from build123d import *

# Parameters (mm, degrees)
CROQUIS1_R                                           = 42.5
CROQUIS1_R_2                                         = 12.5
SALIENTE_EXTRUIR1_DEPTH                              = 7
REFRENTADO_PARA_TORNILLO_TAP_N_CON_CABEZ_D           = 6.6
REFRENTADO_PARA_TORNILLO_TAP_N_CON_CABEZ_DEPTH       = 10
REFRENTADO_PARA_TORNILLO_TAP_N_CON_CABEZ_CSINK_D     = 13.44
REFRENTADO_PARA_TORNILLO_TAP_N_CON_CABEZ_CSINK_ANGLE = 90
REFRENTADO_PARA_TORNILLO_TAP_N_CON_CABEZ_TIP         = 1.982840043
REFRENTADO_PARA_TORNILLO_CON_CABEZA_TRON_D           = 3.4
REFRENTADO_PARA_TORNILLO_CON_CABEZA_TRON_DEPTH       = 10
REFRENTADO_PARA_TORNILLO_CON_CABEZA_TRON_CBORE_D     = 7
REFRENTADO_PARA_TORNILLO_CON_CABEZA_TRON_CBORE_DEPTH = 2.4
REFRENTADO_PARA_TORNILLO_CON_CABEZA_TRON_TIP         = 1.021463052


with BuildPart() as part:
    # Croquis1 → Saliente-Extruir1 (new body)
    with BuildSketch(Plane.XY):
        Circle(CROQUIS1_R)
        Circle(CROQUIS1_R_2, mode=Mode.SUBTRACT)
    extrude(amount=SALIENTE_EXTRUIR1_DEPTH)

    # Refrentado para tornillo tapón con cabeza plana de clavija de M61
    with Locations(Plane.XY.offset(7)):
        with Locations((0, 25), (17.67766953, 17.67766953), (25, 0), (17.67766953, -17.67766953), (0, -25), (-17.67766953, -17.67766953), (-25, 0), (-17.67766953, 17.67766953)):
            CounterSinkHole(REFRENTADO_PARA_TORNILLO_TAP_N_CON_CABEZ_D / 2, REFRENTADO_PARA_TORNILLO_TAP_N_CON_CABEZ_CSINK_D / 2, depth=REFRENTADO_PARA_TORNILLO_TAP_N_CON_CABEZ_DEPTH, counter_sink_angle=REFRENTADO_PARA_TORNILLO_TAP_N_CON_CABEZ_CSINK_ANGLE)
            with Locations((0, 0, -(REFRENTADO_PARA_TORNILLO_TAP_N_CON_CABEZ_DEPTH + REFRENTADO_PARA_TORNILLO_TAP_N_CON_CABEZ_TIP / 2))):  # 118° drill point
                Cone(0, REFRENTADO_PARA_TORNILLO_TAP_N_CON_CABEZ_D / 2, REFRENTADO_PARA_TORNILLO_TAP_N_CON_CABEZ_TIP, mode=Mode.SUBTRACT)

    # Refrentado para tornillo con cabeza troncocónica de M32
    with Locations(Plane(origin=(0, 0, 0), x_dir=(-1, 0, 0), z_dir=(0, 0, -1))):
        with Locations((0, 35), (24.748737342, 24.748737342), (35, 0), (24.748737342, -24.748737342), (0, -35), (-24.748737342, -24.748737342), (-35, 0), (-24.748737342, 24.748737342)):
            CounterBoreHole(REFRENTADO_PARA_TORNILLO_CON_CABEZA_TRON_D / 2, REFRENTADO_PARA_TORNILLO_CON_CABEZA_TRON_CBORE_D / 2, REFRENTADO_PARA_TORNILLO_CON_CABEZA_TRON_CBORE_DEPTH, depth=REFRENTADO_PARA_TORNILLO_CON_CABEZA_TRON_DEPTH)
            with Locations((0, 0, -(REFRENTADO_PARA_TORNILLO_CON_CABEZA_TRON_DEPTH + REFRENTADO_PARA_TORNILLO_CON_CABEZA_TRON_TIP / 2))):  # 118° drill point
                Cone(0, REFRENTADO_PARA_TORNILLO_CON_CABEZA_TRON_D / 2, REFRENTADO_PARA_TORNILLO_CON_CABEZA_TRON_TIP, mode=Mode.SUBTRACT)


solid = part.part
Input: part model. Units: mm. Frame: model coordinates. A direction names the side the tool comes from. Give positions to 0.01 mm unless a question says otherwise; leave off trailing zeros. Write each loop counter-clockwise with the first axis right and the second up, starting at its lowest first coordinate (ties: lowest second). Pieces come first, ordered by that corner, then holes. Notation, with made-up numbers: M 49,47 L 104,47 A21 cw 104,82 Z; hole C -9,25.5 d11. An arc over 180 degrees is marked long. Write item = value, one per line. Start each with the question number.
1) First-contact query: pin 1 Ø3 at (x, y) = (0, -35) entering from +Z; pin 2 Ø2 at (x, y) = (23.5, -24) entering from -Z; pin 3 Ø4 at (y, z) = (-24, 2) entering from +X; pin 4 Ø3 at (y, z) = (32, 6) entering from +X. Flat tips, straight axial feed; report the tip coordinate or a pass-through.
2) Reachability of faces 4 (the cylindrical face through (-21.252, -24.595, 1.183)), 5 (the conical face through (16.08, 14.6, 3.75)) from +Z, -Z, +X, -X, +Y, -Y: full face, straight path, thin tool, end or side. Return the list, or none.
3) Material intervals for line 1 along Y through (x, z) = (-18.5, 1.5); line 2 along X through (y, z) = (-24.5, 1.75); line 3 along Y through (x, z) = (0, 3), sorted ascending. Write a range as [from, to].
4) Cut plane B-B on z = 1. Count the separate pieces of the cut face and the enclosed holes in it, then the cut area to 3 significant figures.
5) Cut plane A-A on x = 35. Return the cut outline in (y, z).
6) Draft query along X for faces 1 (the flat face through (9, -9, 0)), 2 (the cylindrical face through (-36.35, -1.03, 4.73)), 3 (the cylindrical face through (-33.727, -25.861, 3.451)). Return one class per face: +X half, -X half, draft (parallel to the pull), parting line (faces both ways), or undercut.
Solved:
q1.pin_1 = through
q1.pin_2 = 2.4
q1.pin_3 = 36.36
q1.pin_4 = 29.6
q2.face_4 = -Z
q2.face_5 = +Z
q3.line_1 = [-38.26, -20.87], [-14.48, 14.48], [20.87, 38.26]
q3.line_2 = [-34.73, -28.24], [-21.26, -3.26], [3.26, 21.26], [28.24, 34.73]
q3.line_3 = [-42.5, -36.7], [-33.3, -28.3], [-21.7, -12.5], [12.5, 21.7], [28.3, 33.3], [36.7, 42.5]
q4.separate_pieces = 1
q4.enclosed_holes = 17
q4.area = 4,600 mm2
q5.outline = M -24.11,0 L -3.5,0 L -3.5,2.4 L -1.7,2.4 L -1.7,7 L -24.11,7 Z; M 1.7,2.4 L 3.5,2.4 L 3.5,0 L 24.11,0 L 24.11,7 L 1.7,7 Z
q6.face_1 = draft
q6.face_2 = undercut
q6.face_3 = parting line
